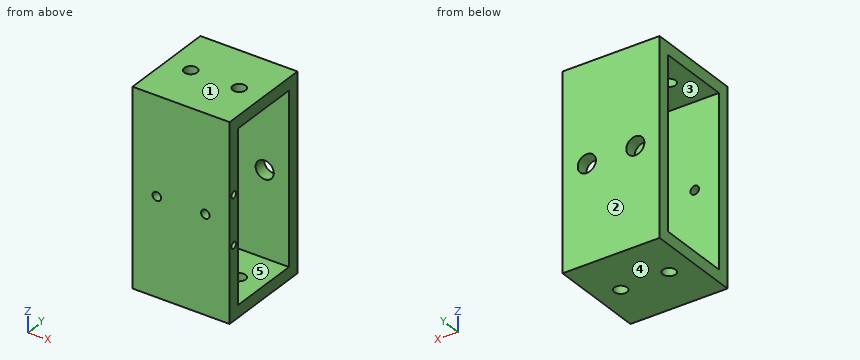
```python
from build123d import *

# Parameters (mm, degrees)
SKETCH2_W                        = 101.6
SKETCH2_H                        = 50.8
SKETCH2_W_2                      = 88.9
SKETCH2_H_2                      = 38.1
BOSS_EXTRUDE1_DEPTH              = 25.4
F_1_4_CLEARANCE_HOLE1_D          = 6.7564
F_8_CLEARANCE_HOLE1_D            = 4.4958
F_8_CLEARANCE_HOLE1_DEPTH        = 6.35
F_3_8_0_375_DIAMETER_HOLE1_D     = 9.525
F_3_8_0_375_DIAMETER_HOLE1_DEPTH = 6.35
F_8_32_TAPPED_HOLE1_D            = 3.4544
F_8_32_TAPPED_HOLE1_DEPTH        = 12.7
F_8_32_TAPPED_HOLE1_TIP          = 1.037806461


with BuildPart() as part:
    # Sketch2 → Boss-Extrude1 (new body, symmetric)
    with BuildSketch(Plane(origin=(0, 0, 0), x_dir=(0, 0, -1), z_dir=(1, 0, 0))):
        Rectangle(SKETCH2_W, SKETCH2_H)
        Rectangle(SKETCH2_W_2, SKETCH2_H_2, mode=Mode.SUBTRACT)
    extrude(amount=BOSS_EXTRUDE1_DEPTH, both=True)

    # 1/4 Clearance Hole1 (through all)
    with Locations(Plane.XY.offset(50.8)):
        with Locations((-12.7, 0), (12.7, 0)):
            Hole(F_1_4_CLEARANCE_HOLE1_D / 2)

    # #8 Clearance Hole1
    with Locations(Plane(origin=(0, -19.05, 0), x_dir=(1, 0, 0), z_dir=(0, 1, 0))):
        with Locations((12.7, 0)):
            f_8_clearance_hole1 = Hole(F_8_CLEARANCE_HOLE1_D / 2, depth=F_8_CLEARANCE_HOLE1_DEPTH)

    # Mirror1: #8 Clearance Hole1 across plane
    add(f_8_clearance_hole1.mirror(Plane(origin=(0, 0, 0), x_dir=(0, 0, 1), z_dir=(1, 0, 0))), mode=Mode.SUBTRACT)

    # 3/8 (0.375) Diameter Hole1
    with Locations(Plane(origin=(0, 25.4, 0), x_dir=(1, 0, 0), z_dir=(0, 1, 0))):
        with Locations((-12.7, 0), (12.7, 0)):
            Hole(F_3_8_0_375_DIAMETER_HOLE1_D / 2, depth=F_3_8_0_375_DIAMETER_HOLE1_DEPTH)

    # #8-32 Tapped Hole1
    with Locations(Plane(origin=(25.4, 0, 0), x_dir=(0, 0, 1), z_dir=(1, 0, 0))):
        with Locations((-12.7, 22.225), (12.7, 22.225)):
            Hole(F_8_32_TAPPED_HOLE1_D / 2, depth=F_8_32_TAPPED_HOLE1_DEPTH)
            with Locations((0, 0, -(F_8_32_TAPPED_HOLE1_DEPTH + F_8_32_TAPPED_HOLE1_TIP / 2))):  # 118° drill point
                Cone(0, F_8_32_TAPPED_HOLE1_D / 2, F_8_32_TAPPED_HOLE1_TIP, mode=Mode.SUBTRACT)


solid = part.part
```
Here's how the part is built. I have some questions about the finished solid (model axes, mm). Face numbers are marked on the shaded views. A direction names the side the tool comes from. Coordinates: 2 decimals unless noted, no trailing zeros. Loops run counter-clockwise (first coordinate to the right, second up) from the corner with the lowest first, then second, coordinate; pieces in that order, holes last. Notation, with made-up numbers: (10, 32) - (58, 32) arc R16 cw to (58, 55) - close; hole circle Ø8 at (-13.75, -39.5). An arc over 180 degrees is marked (long way). Answer as CSV lines item,"result".
Q1. For pin 1 (8.5 mm diameter, centred on x = -12.7, z = 0, fed in from +Y); pin 2 (2 mm diameter, centred on y = -22.225, z = 12.7, fed in from +X), each with a flat end and sliding along its axis, tell me the tip position at first contact or that it passes through.
Response:
pin 1,"y = -19.05"
pin 2,"x = 12.26"
Q2. If we section it at C-C, the plane y = 0: Write out the boundary of the cut face in (x, z), and give its area (3 significant figures).
Response:
outline,"(-25.4, -50.8) - (-16.08, -50.8) - (-16.08, -44.45) - (-25.4, -44.45) - close; (-25.4, 44.45) - (-16.08, 44.45) - (-16.08, 50.8) - (-25.4, 50.8) - close; (-9.32, -50.8) - (9.32, -50.8) - (9.32, -44.45) - (-9.32, -44.45) - close; (-9.32, 44.45) - (9.32, 44.45) - (9.32, 50.8) - (-9.32, 50.8) - close; (16.08, -50.8) - (25.4, -50.8) - (25.4, -44.45) - (16.08, -44.45) - close; (16.08, 44.45) - (25.4, 44.45) - (25.4, 50.8) - (16.08, 50.8) - close"
area,"474 mm2"
Q3. If we section it at A-A, the plane y = 8.5: Write out the boundary of the cut face in (x, z), and give its area (3 significant figures).
Response:
outline,"(-25.4, -50.8) - (25.4, -50.8) - (25.4, -44.45) - (-25.4, -44.45) - close; (-25.4, 44.45) - (25.4, 44.45) - (25.4, 50.8) - (-25.4, 50.8) - close"
area,"645 mm2"
Q4. For the marked faces 4 and 5, which set-ups out of +Z, -Z, +X, -X, +Y, -Y let a thin tool reach every point of the face, with its end or its side?
Response:
face 4,"-Z, +X, -X, +Y, -Y"
face 5,"+X, -X"
Q5. If we section it at D-D, the plane z = 0: Write out the boundary of the cut face in (x, y).
Response:
outline,"(-25.4, -25.4) - (-14.95, -25.4) - (-14.95, -19.05) - (-25.4, -19.05) - close; (-25.4, 19.05) - (-17.46, 19.05) - (-17.46, 25.4) - (-25.4, 25.4) - close; (-10.45, -25.4) - (10.45, -25.4) - (10.45, -19.05) - (-10.45, -19.05) - close; (-7.94, 19.05) - (7.94, 19.05) - (7.94, 25.4) - (-7.94, 25.4) - close; (14.95, -25.4) - (25.4, -25.4) - (25.4, -19.05) - (14.95, -19.05) - close; (17.46, 19.05) - (25.4, 19.05) - (25.4, 25.4) - (17.46, 25.4) - close"
Q6. If we section it at B-B, the plane x = -3.5: Write out the boundary of the cut face in (y, z).
Response:
outline,"(-25.4, -50.8) - (25.4, -50.8) - (25.4, 50.8) - (-25.4, 50.8) - close; hole (-19.05, -44.45) - (19.05, -44.45) - (19.05, 44.45) - (-19.05, 44.45) - close"
Q7. If I drill on L1, parallel to Y at x = -5, z = 4.5; L2, parallel to Z at x = -6, y = 2; L3, parallel to Z at x = 12.7, y = -21.25, over which ranges is the centre line in solid material (lowest first)? Write a range as [from, to].
Response:
L1,"[-25.4, -19.05], [19.05, 25.4]"
L2,"[-50.8, -44.45], [44.45, 50.8]"
L3,"[-50.8, -14.13], [-11.27, -2.25], [2.25, 11.27], [14.13, 50.8]"
Q8. We'd pull the mould along Y, two halves only. Please class the marked faces 1, 2 and 3: pulls with the +Y half, pulls with the -Y half, needs draft (parallel to the pull), parting line crosses it, or undercut.
Response:
face 1,"needs draft"
face 2,"pulls with the +Y half"
face 3,"undercut"
